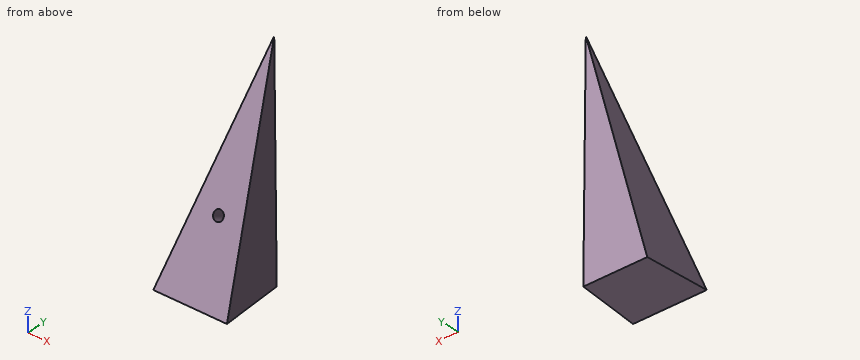
```python
from build123d import *

# Parameters (mm, degrees)
F1_DEPTH = 50.8
F3_DEPTH = 61.1638386197
F4_R     = 3.4925
F5_DEPTH = 28.37362


with BuildPart() as f1:
    # F0 (on Right) → F1 (new body)
    with BuildSketch(Plane.YZ):
        Polygon((46.165614252, 136.1587293462), (-22.2928433907, 0), (22.1571566093, 0), align=None)
    extrude(amount=F1_DEPTH)

    # F2 (on face) → F3 (cut, through all)
    with BuildSketch(Plane(origin=(0, -17.7945295552, 8.9468082853), x_dir=(1, 0, 0), z_dir=(0, -0.8934299826, 0.449202478))):
        Polygon((0, 142.3859995079), (0, -10.0140004921), (25.4, 142.3859995079), align=None)
        Polygon((50.8, 142.3859995079), (25.4, 142.3859995079), (50.8, -10.0140004921), align=None)
    extrude(amount=-F3_DEPTH, mode=Mode.SUBTRACT)

    # F4 (on face) → F5 (cut)
    with BuildSketch(Plane(origin=(0, -17.7945295552, 8.9468082853), x_dir=(1, 0, 0), z_dir=(0, -0.8934299826, 0.449202478))):
        with Locations((25.4, 41.371035104)):
            Circle(F4_R)
    extrude(amount=-F5_DEPTH, mode=Mode.SUBTRACT)


solid = f1.part
```
Could you check a few things on this model? Use its own coordinates, in mm. Round coordinates to 2 decimals unless told otherwise and drop trailing zeros. Loops run counter-clockwise (first coordinate to the right, second up) from the corner with the lowest first, then second, coordinate; pieces in that order, holes last. Notation, with made-up numbers: (-26.75, 77) - (2.25, 77) arc R26 ccw to (2.25, 94) - close; hole circle Ø10 at (-37, -6.5). An arc over 180 degrees is marked (long way). Answer in a Markdown table with one row per item. Add a question column.
(1) If we section it at A-A (x = 24): Please give me the cut outline in (y, z), plus the area to 3 significant figures.
(2) I'm going to push flat-ended pins straight in: pin 1 (3 mm diameter, centred on x = 31.5, y = -11, fed in from +Z); pin 2 (1 mm diameter, centred on y = 24, z = 97.5, fed in from +X); pin 3 (8 mm diameter, centred on x = 7, z = 22.5, fed in from -Y); pin 4 (1 mm diameter, centred on x = 29.5, z = 45, fed in from +Y). Where does each tip first touch, or does it pass through?
(3) If we section it at B-B (y = 29): Please give me the cut outline in (x, z), plus the area to 3 significant figures.
(4) If we section it at C-C (z = 119): Please give me the cut outline in (x, y).
(5) I need wall thicknesses on line 1 along Z through (x, y) = (28.5, 3.5); line 2 along Z through (x, y) = (8.5, -5); line 3 along Z through (x, y) = (27, -0.5). Which ranges of each line are inside material? Lowest first, please.
Model answer:
| question | item | result |
|---|---|---|
| 1 | outline | (-22.29, 0) - (22.16, 0) - (44.64, 127.52) - (42.39, 128.65) - (2.23, 48.77) - (27.58, 36.02) - (24.7, 30.3) - (-0.65, 43.05) - close |
| 1 | area | 2,830 mm² |
| 2 | pin 1 | stops at z = 25.44 |
| 2 | pin 2 | passes through |
| 2 | pin 3 | stops at y = -12.99 |
| 2 | pin 4 | stops at y = 30.18 |
| 3 | outline | (9.62, 38.81) - (41.18, 38.81) - (31.77, 102.02) - (19.03, 102.02) - close |
| 3 | area | 1,400 mm² |
| 4 | outline | (22.2, 37.54) - (28.6, 37.54) - (28.18, 43.14) - (22.62, 43.14) - close |
| 5 | line 1 | z = 0 to 42.75, 46.35 to 51.3 |
| 5 | line 2 | z = 0 to 34.39 |
| 5 | line 3 | z = 0 to 43.08 |
